Design review of the part built by this model. Coordinates are the model's own, in mm. Face numbers are marked on the shaded views. Round coordinates to 2 decimals unless told otherwise and drop trailing zeros. Order: outer loops, then holes, each group sorted by start corner. A loop starts at its lowest first (then second) coordinate and runs counter-clockwise, first axis right, second up. Notation, with made-up numbers: M 8,-9.5 L 64,-9.5 A22 ccw 64,20.5 Z; hole C -14,15.5 d9. An arc over 180 degrees is marked long. Use a Markdown table: item, result. Add a question column.
(1) Take a section at C-C (y = -4). Count the separate pieces of the cut face and the enclosed holes in it, then the cut area to 3 significant figures.
(2) Take a section at A-A (y = 26). Write out the cut boundary in (x, z), then the cut area to 3 significant figures.
(3) For pin 1 (2 mm diameter, centred on x = 6, z = 4, fed in from -Y); pin 2 (1.5 mm diameter, centred on x = 25, z = 3, fed in from +Y); pin 3 (3 mm diameter, centred on x = -9, z = -0.5, fed in from -Y), all flat-tipped, find the tip position at first contact; note any pin that passes through.
(4) The part is to be moulded in two halves that separate along Y. For the marked faces 1 and 2, say which applies: released by +Y, released by -Y, zero draft, split by the parting line, or undercut.
(5) Take a section at B-B (y = -13). Write out the cut boundary in (x, z), then the cut area to 3 significant figures.
(6) To check wall thickness, follow probe 1 along X at (y, z) = (-12.5, -3); probe 2 along X at (y, z) = (-6.5, -2.5); probe 3 along Y at (x, z) = (-13, 2). State the ranges of each line that lie inside material, in increasing order. Write a range as from..to.
```python
from build123d import *

# Parameters (mm, degrees)
F0_R          = 11
F1_DEPTH      = 3.5
F2_R          = 11
F3_DEPTH      = 3.501
F3_DEPTH_BACK = 3.501
F4_T2_ANGLE   = 240
F4_T4_ANGLE   = 240
F4_T6_ANGLE   = 120
F4_T8_ANGLE   = 120
F4_T10_ANGLE  = 240
F4_T12_ANGLE  = 240
F4_T14_ANGLE  = 120
F4_T16_ANGLE  = 120
F4_T18_ANGLE  = 240
F4_T20_ANGLE  = 240
F4_T22_ANGLE  = 120
F4_T24_ANGLE  = 120
F5_R          = 13.8452994616
F5_R_2        = 11
F6_DEPTH      = 2


# Not quite as in the source:
# - a fillet or chamfer that OpenCascade refuses, or shapes differently, is made with other operations: its cross-section is extruded or revolved along the edge and cut away or added


with BuildPart() as f1:
    # F0 (on Top) → F1 (new body, symmetric)
    with BuildSketch(Plane.XY):
        with BuildLine():
            ThreePointArc((-22.5166604984, 2), (-35.5070415552, -20.5), (-9.5262794416, -20.5))
            ThreePointArc((-9.5262794416, -20.5), (0, -15), (9.5262794416, -20.5))
            ThreePointArc((9.5262794416, -20.5), (35.5070415552, -20.5), (22.5166604984, 2))
            ThreePointArc((22.5166604984, 2), (12.9903810568, 7.5), (12.9903810568, 18.5))
            ThreePointArc((12.9903810568, 18.5), (0, 41), (-12.9903810568, 18.5))
            ThreePointArc((-12.9903810568, 18.5), (-12.9903810568, 7.5), (-22.5166604984, 2))
        make_face()
        with Locations((-22.5166604984, -13)):
            Circle(F0_R, mode=Mode.SUBTRACT)
        with Locations((22.5166604984, -13)):
            Circle(F0_R, mode=Mode.SUBTRACT)
        Circle(F0_R, mode=Mode.SUBTRACT)
        with Locations((0, 26)):
            Circle(F0_R, mode=Mode.SUBTRACT)
    extrude(amount=F1_DEPTH, both=True)

    # F2 (on Top) → F3 (cut, two sides)
    with BuildSketch(Plane.XY) as f3_sk:
        Circle(F2_R)
    extrude(amount=-F3_DEPTH, mode=Mode.SUBTRACT)
    extrude(f3_sk.sketch, amount=F3_DEPTH_BACK, mode=Mode.SUBTRACT)

    # F4: chamfer of 2 x 1.1547005384 on 12 edges, made by hand

    # F4_s1 → F4_t2 (revolve, cut)
    with BuildSketch(Plane.YZ.offset(-22.5166604984)):
        Polygon((0.8452994616, 3.5), (2, 1.5), (2, 3.5), align=None)
    revolve(axis=Axis((-22.5166604984, -13, 3.5), (0, 0, 1)), revolution_arc=F4_T2_ANGLE, mode=Mode.SUBTRACT)

    # F4_s3 → F4_t4 (revolve, cut)
    with BuildSketch(Plane.YZ.offset(-22.5166604984)):
        Polygon((2, -1.5), (0.8452994616, -3.5), (2, -3.5), align=None)
    revolve(axis=Axis((-22.5166604984, -13, -3.5), (0, 0, 1)), revolution_arc=F4_T4_ANGLE, mode=Mode.SUBTRACT)

    # F4_s5 → F4_t6 (revolve, cut)
    with BuildSketch(Plane(origin=(-11.2583302492, 19.5, 0), x_dir=(0, 0, 1), z_dir=(-0.5, 0.8660254038, 0))):
        Polygon((-1.5, -2), (-3.5, -0.8452994616), (-3.5, -2), align=None)
    revolve(axis=Axis((-22.5166604984, 13, -3.5), (0, 0, -1)), revolution_arc=F4_T6_ANGLE, mode=Mode.SUBTRACT)

    # F4_s7 → F4_t8 (revolve, cut)
    with BuildSketch(Plane(origin=(-11.2583302492, 19.5, 0), x_dir=(0, 0, 1), z_dir=(-0.5, 0.8660254038, 0))):
        Polygon((1.5, -2), (3.5, -0.8452994616), (3.5, -2), align=None)
    revolve(axis=Axis((-22.5166604984, 13, 3.5), (0, 0, -1)), revolution_arc=F4_T8_ANGLE, mode=Mode.SUBTRACT)

    # F4_s9 → F4_t10 (revolve, cut)
    with BuildSketch(Plane(origin=(11.2583302492, 19.5, 0), x_dir=(0, 0, 1), z_dir=(-0.5, -0.8660254038, 0))):
        Polygon((-1.5, -2), (-3.5, -0.8452994616), (-3.5, -2), align=None)
    revolve(axis=Axis((0, 26, -3.5), (0, 0, 1)), revolution_arc=F4_T10_ANGLE, mode=Mode.SUBTRACT)

    # F4_s11 → F4_t12 (revolve, cut)
    with BuildSketch(Plane(origin=(11.2583302492, 19.5, 0), x_dir=(0, 0, 1), z_dir=(-0.5, -0.8660254038, 0))):
        Polygon((1.5, -2), (3.5, -0.8452994616), (3.5, -2), align=None)
    revolve(axis=Axis((0, 26, 3.5), (0, 0, 1)), revolution_arc=F4_T12_ANGLE, mode=Mode.SUBTRACT)

    # F4_s13 → F4_t14 (revolve, cut)
    with BuildSketch(Plane.YZ.offset(22.5166604984)):
        Polygon((2, -1.5), (0.8452994616, -3.5), (2, -3.5), align=None)
    revolve(axis=Axis((22.5166604984, 13, -3.5), (0, 0, -1)), revolution_arc=F4_T14_ANGLE, mode=Mode.SUBTRACT)

    # F4_s15 → F4_t16 (revolve, cut)
    with BuildSketch(Plane.YZ.offset(22.5166604984)):
        Polygon((2, 1.5), (0.8452994616, 3.5), (2, 3.5), align=None)
    revolve(axis=Axis((22.5166604984, 13, 3.5), (0, 0, -1)), revolution_arc=F4_T16_ANGLE, mode=Mode.SUBTRACT)

    # F4_s17 → F4_t18 (revolve, cut)
    with BuildSketch(Plane(origin=(11.2583302492, -19.5, 0), x_dir=(0, 0, 1), z_dir=(-0.5, 0.8660254038, 0))):
        Polygon((-1.5, -2), (-3.5, -0.8452994616), (-3.5, -2), align=None)
    revolve(axis=Axis((22.5166604984, -13, -3.5), (0, 0, 1)), revolution_arc=F4_T18_ANGLE, mode=Mode.SUBTRACT)

    # F4_s19 → F4_t20 (revolve, cut)
    with BuildSketch(Plane(origin=(11.2583302492, -19.5, 0), x_dir=(0, 0, 1), z_dir=(-0.5, 0.8660254038, 0))):
        Polygon((1.5, -2), (3.5, -0.8452994616), (3.5, -2), align=None)
    revolve(axis=Axis((22.5166604984, -13, 3.5), (0, 0, 1)), revolution_arc=F4_T20_ANGLE, mode=Mode.SUBTRACT)

    # F4_s21 → F4_t22 (revolve, cut)
    with BuildSketch(Plane(origin=(-11.2583302492, -19.5, 0), x_dir=(0, 0, 1), z_dir=(-0.5, -0.8660254038, 0))):
        Polygon((-1.5, -2), (-3.5, -0.8452994616), (-3.5, -2), align=None)
    revolve(axis=Axis((0, -26, -3.5), (0, 0, -1)), revolution_arc=F4_T22_ANGLE, mode=Mode.SUBTRACT)

    # F4_s23 → F4_t24 (revolve, cut)
    with BuildSketch(Plane(origin=(-11.2583302492, -19.5, 0), x_dir=(0, 0, 1), z_dir=(-0.5, -0.8660254038, 0))):
        Polygon((1.5, -2), (3.5, -0.8452994616), (3.5, -2), align=None)
    revolve(axis=Axis((0, -26, 3.5), (0, 0, -1)), revolution_arc=F4_T24_ANGLE, mode=Mode.SUBTRACT)

    # F5 (on face) → F6 (join)
    with BuildSketch(Plane.XY.offset(3.5)):
        Circle(F5_R)
        Circle(F5_R_2, mode=Mode.SUBTRACT)
    extrude(amount=F6_DEPTH)


solid = f1.part
```
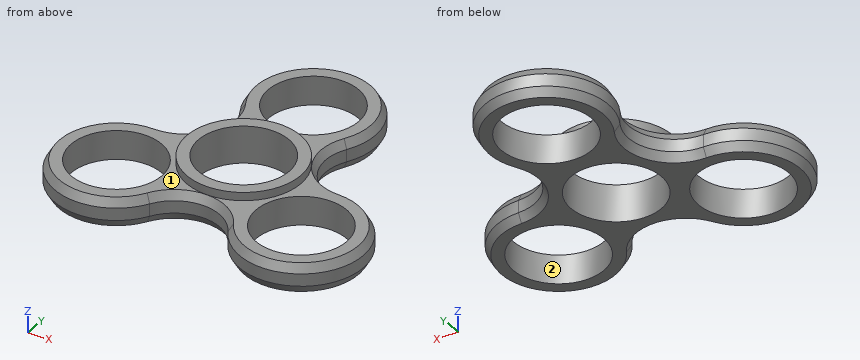
Verdict:
| question | item | result |
|---|---|---|
| 1 | separate pieces | 4 |
| 1 | enclosed holes | 0 |
| 1 | area | 169 mm^2 |
| 2 | outline | M -15,-1.5 L -13.85,-3.5 L -11,-3.5 L -11,3.5 L -13.85,3.5 L -15,1.5 Z; M 11,-3.5 L 13.85,-3.5 L 15,-1.5 L 15,1.5 L 13.85,3.5 L 11,3.5 Z |
| 2 | area | 51.4 mm^2 |
| 3 | pin 1 | stops at y = -16.01 |
| 3 | pin 2 | stops at y = 1.37 |
| 3 | pin 3 | stops at y = -21.98 |
| 4 | face 1 | zero draft |
| 4 | face 2 | undercut |
| 5 | outline | M -37.52,-1.5 L -36.36,-3.5 L -33.52,-3.5 L -33.52,3.5 L -36.36,3.5 L -37.52,1.5 Z; M -11.52,-3.5 L 11.52,-3.5 L 11.52,3.5 L 4.76,3.5 L 4.76,5.5 L -4.76,5.5 L -4.76,3.5 L -11.52,3.5 Z; M 33.52,-3.5 L 36.36,-3.5 L 37.52,-1.5 L 37.52,1.5 L 36.36,3.5 L 33.52,3.5 Z |
| 5 | area | 232 mm^2 |
| 6 | probe 1 | x = -36.64..-33.51, -11.53..11.53, 33.51..36.64 |
| 6 | probe 2 | x = -35.39..-31.39, -13.64..-8.87, 8.87..13.64, 31.39..35.39 |
| 6 | probe 3 | y = -24.22..-18.52, -7.48..6.93, 19.11..32.89 |
